Geometry check sheet. Reference: the model listing, model coordinates, mm. Round coordinates to 2 decimals unless told otherwise and drop trailing zeros. Write each loop counter-clockwise with the first axis right and the second up, starting at its lowest first coordinate (ties: lowest second). Pieces come first, ordered by that corner, then holes. Notation, with made-up numbers: M 26.5,-36 L 79.5,-36 A15 ccw 79.5,-14 Z; hole C -38.75,53 d7. An arc over 180 degrees is marked long. Use a Markdown table: item, result.
```python
from build123d import *

# Parameters (mm, degrees)
SKETCH1_R          = 127
BASE_DEPTH         = 5.334
SKETCH2_R          = 76.2
CENTER_CUT_DEPTH   = 180.684310823
SKETCH14_W         = 5
SKETCH14_H         = 6.35
SKETCH14_W_2       = 6.35
SKETCH14_H_2       = 5
CUT_EXTRUDE1_DEPTH = 180.684310823
SKETCH15_W         = 30.48
SKETCH15_H         = 48.26
CUT_EXTRUDE2_DEPTH = 180.684310823
HOLE1_OUTLINE_R    = 3.175
HOLE1_DEPTH        = 5.334


# Read off the part's stored shape, not the designer's step: Hole1
with BuildPart() as part:
    # Sketch1 → Base (new body)
    with BuildSketch(Plane(origin=(0, 0, 0), x_dir=(1, 0, 0), z_dir=(0, 1, 0))):
        with Locations(Location((0, 0, 0), (0, 0, 270))):
            Circle(SKETCH1_R)
    extrude(amount=BASE_DEPTH)

    # Sketch2 → Center Cut (cut, through all)
    with BuildSketch(Plane(origin=(0, 5.334, 0), x_dir=(1, 0, 0), z_dir=(0, 1, 0))):
        with Locations(Location((0, 0, 0), (0, 0, 270))):
            Circle(SKETCH2_R)
    extrude(amount=-CENTER_CUT_DEPTH, mode=Mode.SUBTRACT)

    # Sketch14 → Cut-Extrude1 (cut, through all)
    with BuildSketch(Plane.XZ):
        with Locations((0, 89.789)):
            Rectangle(SKETCH14_W, SKETCH14_H)
        with Locations((-17.78, 89.789)):
            Rectangle(SKETCH14_W, SKETCH14_H)
        with Locations((17.78, 89.789)):
            Rectangle(SKETCH14_W, SKETCH14_H)
        with Locations((-80.899, -26.63)):
            Rectangle(SKETCH14_W_2, SKETCH14_H_2)
        with Locations((-80.899, -43.06)):
            Rectangle(SKETCH14_W_2, SKETCH14_H_2)
        with Locations((-80.899, -59.49)):
            Rectangle(SKETCH14_W_2, SKETCH14_H_2)
        with Locations((80.899, -26.63)):
            Rectangle(SKETCH14_W_2, SKETCH14_H_2)
        with Locations((80.899, -43.06)):
            Rectangle(SKETCH14_W_2, SKETCH14_H_2)
        with Locations((80.899, -59.49)):
            Rectangle(SKETCH14_W_2, SKETCH14_H_2)
        with Locations((17.78, -89.789)):
            Rectangle(SKETCH14_W, SKETCH14_H)
        with Locations((0, -89.789)):
            Rectangle(SKETCH14_W, SKETCH14_H)
        with Locations((-17.78, -89.789)):
            Rectangle(SKETCH14_W, SKETCH14_H)
    extrude(amount=-CUT_EXTRUDE1_DEPTH, mode=Mode.SUBTRACT)

    # Sketch15 → Cut-Extrude2 (cut, through all)
    with BuildSketch(Plane.XZ):
        with Locations((-116.84, 0)):
            Rectangle(SKETCH15_W, SKETCH15_H)
        with Locations((116.84, 0)):
            Rectangle(SKETCH15_W, SKETCH15_H)
    extrude(amount=-CUT_EXTRUDE2_DEPTH, mode=Mode.SUBTRACT)

    # Hole1 outline → Hole1 (cut)
    with BuildSketch(Plane(origin=(0, 0, 0), x_dir=(1, 0, 0), z_dir=(0, 1, 0))):
        with Locations((-54.61, -78.74)):
            Circle(HOLE1_OUTLINE_R)
        with Locations((54.61, -78.74)):
            Circle(HOLE1_OUTLINE_R)
        with Locations((54.61, 78.74)):
            Circle(HOLE1_OUTLINE_R)
        with Locations((-54.61, 78.74)):
            Circle(HOLE1_OUTLINE_R)
    extrude(amount=HOLE1_DEPTH, mode=Mode.SUBTRACT)


solid = part.part
```
Item 1: Cross-section at C-C, the plane y = 4.5. Count the separate pieces of the cut face and the enclosed holes in it, and give its area (3 significant figures).
Outcome:
| item | result |
|---|---|
| separate pieces | 1 |
| enclosed holes | 17 |
| area | 29,500 mm2 |
Item 2: Cross-section at D-D, the plane x = -107. Record the cut outline in (y, z), and give its area (3 significant figures).
Outcome:
| item | result |
|---|---|
| outline | M 0,-68.41 L 5.33,-68.41 L 5.33,-24.13 L 0,-24.13 Z; M 0,24.13 L 5.33,24.13 L 5.33,68.41 L 0,68.41 Z |
| area | 472 mm2 |
Item 3: Cross-section at A-A, the plane z = 0. Record the cut outline in (x, y), and give its area (3 significant figures).
Outcome:
| item | result |
|---|---|
| outline | M -101.6,0 L -76.2,0 L -76.2,5.33 L -101.6,5.33 Z; M 76.2,0 L 101.6,0 L 101.6,5.33 L 76.2,5.33 Z |
| area | 271 mm2 |
Item 4: Mould release check, pull along Z, two halves, no side actions. Record for faces 1 (the face through (-2.453, 2.63, 126.976)), 2 (the face through (57, 0, 55)), 3 (the face through (2.453, 2.63, -126.976)), 4 (the face through (53.92, 2.63, 81.84)): +Z half, -Z half, draft (parallel to the pull), parting line (faces both ways), or undercut.
Outcome:
| item | result |
|---|---|
| face 1 | +Z half |
| face 2 | draft |
| face 3 | -Z half |
| face 4 | undercut |
Item 5: Material ranges on line 1 along X through (y, z) = (1.3, 1.5); line 2 along X through (y, z) = (1.55, -78.74) (3 decimals); line 3 along Z through (x, y) = (54.61, 3.35) (3 decimals), recorded low to high. Write a range as from..to.
Outcome:
| item | result |
|---|---|
| line 1 | x = -101.6..-76.19, 76.19..101.6 |
| line 2 | x = -99.644..-57.785, -51.435..51.435, 57.785..99.644 |
| line 3 | z = -114.659..-81.915, -75.565..-53.143, 53.143..75.565, 81.915..114.659 |
Item 6: Cross-section at B-B, the plane x = 54.61. Record the cut outline in (y, z) (3 decimals), and give its area (3 significant figures).
Outcome:
| item | result |
|---|---|
| outline | M 0,-114.659 L 5.334,-114.659 L 5.334,-81.915 L 0,-81.915 Z; M 0,-75.565 L 5.334,-75.565 L 5.334,-53.143 L 0,-53.143 Z; M 0,53.143 L 5.334,53.143 L 5.334,75.565 L 0,75.565 Z; M 0,81.915 L 5.334,81.915 L 5.334,114.659 L 0,114.659 Z |
| area | 589 mm2 |
Item 7: Go/stop test with flat-tipped pins: pin 1 (2.5 mm diameter, centred on x = -17, y = 2, fed in from -Z); pin 2 (2.5 mm diameter, centred on x = -80.5, y = 4, fed in from +Z); pin 3 (2.5 mm diameter, centred on y = 2, z = 89, fed in from -X). Record where each tip stops, or that it passes through.
Outcome:
| item | result |
|---|---|
| pin 1 | stops at z = -126.02 |
| pin 2 | stops at z = 99.24 |
| pin 3 | stops at x = -91.81 |
